```python
from build123d import *

# Parameters (mm, degrees)
SKETCH1_W           = 84.836
SKETCH1_H           = 8.636
BOSS_EXTRUDE1_DEPTH = 16.256
SKETCH2_W           = 49.276
SKETCH2_H           = 13.97
CUT_EXTRUDE1_DEPTH  = 134.757308654
SKETCH3_R           = 1.778
CUT_EXTRUDE2_DEPTH  = 147.33606739
SKETCH4_W           = 17.018
SKETCH4_H           = 13.716
SKETCH4_W_2         = 13.561760772
SKETCH4_H_2         = 13.376292463
CUT_EXTRUDE3_DEPTH  = 134.757308654


with BuildPart() as part:
    # Sketch1 → Boss-Extrude1 (new body)
    with BuildSketch(Plane(origin=(0, 0, 0), x_dir=(1, 0, 0), z_dir=(0, 1, 0))):
        with Locations((-90.066639058, 55.663726359)):
            Rectangle(SKETCH1_W, SKETCH1_H)
    extrude(amount=BOSS_EXTRUDE1_DEPTH)

    # Sketch2 → Cut-Extrude1 (cut, through all)
    with BuildSketch(Plane.XY.offset(-51.345726359)):
        with Locations((-88.288639058, 6.985)):
            Rectangle(SKETCH2_W, SKETCH2_H)
    extrude(amount=-CUT_EXTRUDE1_DEPTH, mode=Mode.SUBTRACT)

    # Sketch3 → Cut-Extrude2 (cut, through all)
    with BuildSketch(Plane(origin=(0, 16.256, 0), x_dir=(1, 0, 0), z_dir=(0, 1, 0))):
        with Locations(Location((-50.950639058, 55.663726359, 0), (0, 0, 270))):
            Circle(SKETCH3_R)
        with Locations(Location((-125.372639058, 55.663726359, 0), (0, 0, 270))):
            Circle(SKETCH3_R)
    extrude(amount=-CUT_EXTRUDE2_DEPTH, mode=Mode.SUBTRACT)

    # Sketch4 → Cut-Extrude3 (cut, through all)
    with BuildSketch(Plane.XY.offset(-51.345726359)):
        with Locations((-123.975639058, 9.398)):
            Rectangle(SKETCH4_W, SKETCH4_H)
        with Locations((-54.429519444, 9.567853769)):
            Rectangle(SKETCH4_W_2, SKETCH4_H_2)
    extrude(amount=-CUT_EXTRUDE3_DEPTH, mode=Mode.SUBTRACT)


solid = part.part
```
Geometry: final body of the model. Coordinates: model frame, mm. A direction names the side the tool comes from. Coordinates: 2 decimals unless noted, no trailing zeros. Write each loop counter-clockwise with the first axis right and the second up, starting at its lowest first coordinate (ties: lowest second). Pieces come first, ordered by that corner, then holes. Notation, with made-up numbers: M -33.5,4 L -1.5,4 A29 ccw -1.5,36 Z; hole C 9.5,18 d10. An arc over 180 degrees is marked long. Answer as CSV lines item,"result". Start each with the question number.
Q1. Mould query, pull axis X, two halves, no side actions, for faces 1 (the cylindrical face through (-49.19, 1.46, -55.9)), 2 (the flat face through (-123, 0, -56)), 3 (the flat face through (-61.21, 9, -56)). Classes: released by +X, released by -X, zero draft, split by the parting line, or undercut.
Q2. Cut plane C-C on y = 1. Return the cut outline in (x, z), then the cut area to 3 significant figures.
Q3. Cut plane D-D on y = 15.25. Return the cut outline in (x, z), then the cut area to 3 significant figures.
Q4. Pin query (flat end, axial travel): P1, Ø2, axis at y = 12, z = -56.5, coming from the -X side; P2, Ø4.5, axis at y = 6, z = -56, coming from the +X side; P3, Ø2.5, axis at x = -55, z = -56.5, coming from the +Y side; P4, Ø3, axis at x = -125.37, z = -55.66, coming from the -Y side. Return the tip coordinate at first contact, or that it passes through.
Q5. Reachability of faces 4 (the flat face through (-115.467, 9, -56)), 5 (the flat face through (-112.927, 7, -56)), 6 (the flat face through (-55, 2.88, -56)) from +Z, -Z, +X, -X, +Y, -Y: full face, straight path, thin tool, end or side. Return the list, or none.
Q6. Cut plane A-A on y = 8.25. Return the cut outline in (x, z).
Q7. Cut plane B-B on z = -58.25. Return the cut outline in (x, y), then the cut area to 3 significant figures.
Q8. Line query: line 1 (X direction, y = 8, z = -53); line 2 (X direction, y = 2, z = -55); line 3 (Y direction, x = -64.5, z = -55.5). Output: solid intervals per line, ascending. Write a range as from..to.
Findings below:
1,face 1,"undercut"
1,face 2,"zero draft"
1,face 3,"released by +X"
2,outline,"M -132.48,-59.98 L -112.93,-59.98 L -112.93,-51.35 L -132.48,-51.35 Z; M -63.65,-59.98 L -47.65,-59.98 L -47.65,-51.35 L -63.65,-51.35 Z; hole C -125.37,-55.66 d3.56; hole C -50.95,-55.66 d3.56"
2,area,"287 mm2"
3,outline,"M -115.47,-59.98 L -61.21,-59.98 L -61.21,-51.35 L -115.47,-51.35 Z"
3,area,"469 mm2"
4,P1,"stops at x = -115.47"
4,P2,"stops at x = -61.21"
4,P3,"stops at y = 2.88"
4,P4,"passes through"
5,face 4,"+Z, -Z, -X, +Y"
5,face 5,"+Z, -Z, -Y"
5,face 6,"+Z, -Z, +X, +Y"
6,outline,"M -115.47,-59.98 L -112.93,-59.98 L -112.93,-51.35 L -115.47,-51.35 Z; M -63.65,-59.98 L -61.21,-59.98 L -61.21,-51.35 L -63.65,-51.35 Z"
7,outline,"M -132.48,0 L -112.93,0 L -112.93,13.97 L -63.65,13.97 L -63.65,0 L -47.65,0 L -47.65,2.88 L -61.21,2.88 L -61.21,16.26 L -115.47,16.26 L -115.47,2.54 L -132.48,2.54 Z"
7,area,"276 mm2"
8,line 1,"x = -115.47..-112.93, -63.65..-61.21"
8,line 2,"x = -132.48..-127.02, -123.72..-112.93, -63.65..-52.6, -49.3..-47.65"
8,line 3,"y = 13.97..16.26"
